from build123d import *

# Parameters (mm, degrees)
SKETCH_1_R      = 56
SKETCH_1_R_2    = 2.6
SKETCH_1_R_3    = 17.5
SKETCH_1_R_4    = 1.5
EXTRUDE_1_DEPTH = 4
FILLET_1_R      = 3
EXTRUDE_START   = -4
SKETCH_2_R      = 17.5
SKETCH_2_R_2    = 7.5
EXTRUDE_2_DEPTH = 4


with BuildPart() as part:
    # 草图1 → 凸台-拉伸1 (new body)
    with BuildSketch(Plane(origin=(0, 0, 0), x_dir=(1, 0, 0), z_dir=(0, 1, 0))):
        with Locations(Location((0, 0, 0), (0, 0, 270))):
            Circle(SKETCH_1_R)
        with BuildLine():
            Line((-5, 47.236109069), (-5, 27.041634566))
            ThreePointArc((-5, 27.041634566), (-13.75, 23.815698604), (-20.918742494, 17.850944302))
            Line((-20.918742494, 17.850944302), (-38.40767043, 27.948181554))
            ThreePointArc((-38.40767043, 27.948181554), (-23.75, 41.13620668), (-5, 47.236109069))
        make_face(mode=Mode.SUBTRACT)
        with BuildLine():
            Line((-43.40767043, 19.287927516), (-25.918742494, 9.190690264))
            ThreePointArc((-25.918742494, 9.190690264), (-27.5, 0), (-25.918742494, -9.190690264))
            Line((-25.918742494, -9.190690264), (-43.40767043, -19.287927516))
            ThreePointArc((-43.40767043, -19.287927516), (-47.5, 0), (-43.40767043, 19.287927516))
        make_face(mode=Mode.SUBTRACT)
        with BuildLine():
            Line((-38.40767043, -27.948181554), (-20.918742494, -17.850944302))
            ThreePointArc((-20.918742494, -17.850944302), (-13.75, -23.815698604), (-5, -27.041634566))
            Line((-5, -27.041634566), (-5, -47.236109069))
            ThreePointArc((-5, -47.236109069), (-23.75, -41.13620668), (-38.40767043, -27.948181554))
        make_face(mode=Mode.SUBTRACT)
        with BuildLine():
            Line((5, -47.236109069), (5, -27.041634566))
            ThreePointArc((5, -27.041634566), (13.75, -23.815698604), (20.918742494, -17.850944302))
            Line((20.918742494, -17.850944302), (38.40767043, -27.948181554))
            ThreePointArc((38.40767043, -27.948181554), (23.75, -41.13620668), (5, -47.236109069))
        make_face(mode=Mode.SUBTRACT)
        with BuildLine():
            Line((43.40767043, -19.287927516), (25.918742494, -9.190690264))
            ThreePointArc((25.918742494, -9.190690264), (27.5, 0), (25.918742494, 9.190690264))
            Line((25.918742494, 9.190690264), (43.40767043, 19.287927516))
            ThreePointArc((43.40767043, 19.287927516), (47.5, 0), (43.40767043, -19.287927516))
        make_face(mode=Mode.SUBTRACT)
        with BuildLine():
            Line((38.40767043, 27.948181554), (20.918742494, 17.850944302))
            ThreePointArc((20.918742494, 17.850944302), (13.75, 23.815698604), (5, 27.041634566))
            Line((5, 27.041634566), (5, 47.236109069))
            ThreePointArc((5, 47.236109069), (23.75, 41.13620668), (38.40767043, 27.948181554))
        make_face(mode=Mode.SUBTRACT)
        with Locations(Location((0, 22.55, 0), (0, 0, 270))):
            Circle(SKETCH_1_R_2, mode=Mode.SUBTRACT)
        with Locations(Location((-19.528872855, -11.275, 0), (0, 0, 270))):
            Circle(SKETCH_1_R_2, mode=Mode.SUBTRACT)
        with Locations(Location((0, -22.55, 0), (0, 0, 270))):
            Circle(SKETCH_1_R_2, mode=Mode.SUBTRACT)
        with Locations(Location((19.528872855, -11.275, 0), (0, 0, 270))):
            Circle(SKETCH_1_R_2, mode=Mode.SUBTRACT)
        with Locations(Location((-19.528872855, 11.275, 0), (0, 0, 270))):
            Circle(SKETCH_1_R_2, mode=Mode.SUBTRACT)
        with Locations(Location((0, 0, 0), (0, 0, 270))):
            Circle(SKETCH_1_R_3, mode=Mode.SUBTRACT)
        with Locations(Location((19.528872855, 11.275, 0), (0, 0, 270))):
            Circle(SKETCH_1_R_2, mode=Mode.SUBTRACT)
        with Locations(Location((-32.421469697, -40.655237088, 0), (0, 0, 270))):
            Circle(SKETCH_1_R_4, mode=Mode.SUBTRACT)
        with Locations(Location((-40.655237088, -32.421469697, 0), (0, 0, 270))):
            Circle(SKETCH_1_R_4, mode=Mode.SUBTRACT)
        with Locations(Location((-22.561954434, -46.850381131, 0), (0, 0, 270))):
            Circle(SKETCH_1_R_4, mode=Mode.SUBTRACT)
        with Locations(Location((-11.571088566, -50.696251433, 0), (0, 0, 270))):
            Circle(SKETCH_1_R_4, mode=Mode.SUBTRACT)
        with Locations(Location((-46.850381131, -22.561954434, 0), (0, 0, 270))):
            Circle(SKETCH_1_R_4, mode=Mode.SUBTRACT)
        with Locations(Location((-50.696251433, -11.571088566, 0), (0, 0, 270))):
            Circle(SKETCH_1_R_4, mode=Mode.SUBTRACT)
        with Locations(Location((-52, 0, 0), (0, 0, 270))):
            Circle(SKETCH_1_R_4, mode=Mode.SUBTRACT)
        with Locations(Location((0, -52, 0), (0, 0, 270))):
            Circle(SKETCH_1_R_4, mode=Mode.SUBTRACT)
        with Locations(Location((11.571088566, -50.696251433, 0), (0, 0, 270))):
            Circle(SKETCH_1_R_4, mode=Mode.SUBTRACT)
        with Locations(Location((22.561954434, -46.850381131, 0), (0, 0, 270))):
            Circle(SKETCH_1_R_4, mode=Mode.SUBTRACT)
        with Locations(Location((32.421469697, -40.655237088, 0), (0, 0, 270))):
            Circle(SKETCH_1_R_4, mode=Mode.SUBTRACT)
        with Locations(Location((40.655237088, -32.421469697, 0), (0, 0, 270))):
            Circle(SKETCH_1_R_4, mode=Mode.SUBTRACT)
        with Locations(Location((46.850381131, -22.561954434, 0), (0, 0, 270))):
            Circle(SKETCH_1_R_4, mode=Mode.SUBTRACT)
        with Locations(Location((50.696251433, -11.571088566, 0), (0, 0, 270))):
            Circle(SKETCH_1_R_4, mode=Mode.SUBTRACT)
        with Locations(Location((-50.696251433, 11.571088566, 0), (0, 0, 270))):
            Circle(SKETCH_1_R_4, mode=Mode.SUBTRACT)
        with Locations(Location((-46.850381131, 22.561954434, 0), (0, 0, 270))):
            Circle(SKETCH_1_R_4, mode=Mode.SUBTRACT)
        with Locations(Location((-40.655237088, 32.421469697, 0), (0, 0, 270))):
            Circle(SKETCH_1_R_4, mode=Mode.SUBTRACT)
        with Locations(Location((-32.421469697, 40.655237088, 0), (0, 0, 270))):
            Circle(SKETCH_1_R_4, mode=Mode.SUBTRACT)
        with Locations(Location((-22.561954434, 46.850381131, 0), (0, 0, 270))):
            Circle(SKETCH_1_R_4, mode=Mode.SUBTRACT)
        with Locations(Location((-11.571088566, 50.696251433, 0), (0, 0, 270))):
            Circle(SKETCH_1_R_4, mode=Mode.SUBTRACT)
        with Locations(Location((40.655237088, 32.421469697, 0), (0, 0, 270))):
            Circle(SKETCH_1_R_4, mode=Mode.SUBTRACT)
        with Locations(Location((22.561954434, 46.850381131, 0), (0, 0, 270))):
            Circle(SKETCH_1_R_4, mode=Mode.SUBTRACT)
        with Locations(Location((11.571088566, 50.696251433, 0), (0, 0, 270))):
            Circle(SKETCH_1_R_4, mode=Mode.SUBTRACT)
        with Locations(Location((0, 52, 0), (0, 0, 270))):
            Circle(SKETCH_1_R_4, mode=Mode.SUBTRACT)
        with Locations(Location((46.850381131, 22.561954434, 0), (0, 0, 270))):
            Circle(SKETCH_1_R_4, mode=Mode.SUBTRACT)
        with Locations(Location((32.421469697, 40.655237088, 0), (0, 0, 270))):
            Circle(SKETCH_1_R_4, mode=Mode.SUBTRACT)
        with Locations(Location((52, 0, 0), (0, 0, 270))):
            Circle(SKETCH_1_R_4, mode=Mode.SUBTRACT)
        with Locations(Location((50.696251433, 11.571088566, 0), (0, 0, 270))):
            Circle(SKETCH_1_R_4, mode=Mode.SUBTRACT)
    extrude(amount=EXTRUDE_1_DEPTH)

    # 圆角1
    fillet_1_edges = [part.edges().sort_by_distance(p)[0] for p in [
        (5, 2, 27.041634566),
        (5, 2, 47.236109069),
        (38.40767043, 2, 27.948181554),
        (20.918742494, 2, 17.850944302),
        (43.40767043, 2, -19.287927516),
        (25.918742494, 2, -9.190690264),
        (25.918742494, 2, 9.190690264),
        (43.40767043, 2, 19.287927516),
        (5, 2, -47.236109069),
        (5, 2, -27.041634566),
        (20.918742494, 2, -17.850944302),
        (38.40767043, 2, -27.948181554),
        (-38.40767043, 2, -27.948181554),
        (-20.918742494, 2, -17.850944302),
        (-5, 2, -27.041634566),
        (-5, 2, -47.236109069),
        (-43.40767043, 2, 19.287927516),
        (-25.918742494, 2, 9.190690264),
        (-25.918742494, 2, -9.190690264),
        (-43.40767043, 2, -19.287927516),
        (-5, 2, 47.236109069),
        (-5, 2, 27.041634566),
        (-20.918742494, 2, 17.850944302),
        (-38.40767043, 2, 27.948181554),
    ]]
    fillet(fillet_1_edges, radius=FILLET_1_R)

    # 草图2 → 凸台-拉伸2 (add)
    with BuildSketch(Plane(origin=(0, 4, 0), x_dir=(1, 0, 0), z_dir=(0, 1, 0)).offset(EXTRUDE_START)):
        Circle(SKETCH_2_R)
        with Locations(Location((0, 0, 0), (0, 0, 270))):
            Circle(SKETCH_2_R_2, mode=Mode.SUBTRACT)
    extrude(amount=EXTRUDE_2_DEPTH)


solid = part.part
Design review of the part built by this model. Coordinates are the model's own, in mm. Give positions to 0.01 mm unless a question says otherwise; leave off trailing zeros. Loops run counter-clockwise (first coordinate to the right, second up) from the corner with the lowest first, then second, coordinate; pieces in that order, holes last. Notation, with made-up numbers: (-0.5, 2.5) -> (47.5, 2.5) arc R15 ccw to (47.5, 30.5) -> close; hole circle Ø5 at (76, 33.25). An arc over 180 degrees is marked (long way). One line per question, with ' | ' between items. Start each with the question number.
(1) Insertion check: P1, Ø1.5, axis at y = 2, z = 3, coming from the +X side; P2, Ø1.2, axis at y = 2, z = 40, coming from the +X side (3 decimals); P3, Ø2, axis at x = -42, y = 0.5, coming from the +Z side. Each pin has a flat end and moves straight along its axis. Give the tip position at first contact, or say it passes through.
(2) For line 1 (Z direction, x = -35, y = 1.2); line 2 (Z direction, x = -2, y = 2.5); line 3 (X direction, y = 1.35, z = -5.5), list the stretches that pass through material, from the lowest coordinate up.
(3) We need section A-A (z = 0). State the section outline as (x, y) points.
(4) We need section C-C (z = -37). State the section outline as (x, y) points, and give its area (3 significant figures).
(5) We need section D-D (y = 0.6). State how many separate pieces and enclosed holes the cut face has, and give its area (3 significant figures).
(6) We need section B-B (x = 0). State the section outline as (y, z) points, and give its area (3 significant figures).
The answers:
1) P1: stops at x = 55.95 | P2: stops at x = 39.795 | P3: stops at z = 38.14
2) line 1: z = -43.71 to -32.11, -25.98 to -14.43, 14.43 to 25.98, 32.11 to 43.71 | line 2: z = -55.96 to -24.21, -20.89 to -7.23, 7.23 to 20.89, 24.21 to 55.96 | line 3: x = -55.73 to -47.18, -26.94 to -5.1, 5.1 to 26.94, 47.18 to 55.73
3) outline: (-56, 0) -> (-53.5, 0) -> (-53.5, 4) -> (-56, 4) -> close; (-50.5, 0) -> (-47.5, 0) -> (-47.5, 4) -> (-50.5, 4) -> close; (-27.5, 0) -> (-7.5, 0) -> (-7.5, 4) -> (-27.5, 4) -> close; (7.5, 0) -> (27.5, 0) -> (27.5, 4) -> (7.5, 4) -> close; (47.5, 0) -> (50.5, 0) -> (50.5, 4) -> (47.5, 4) -> close; (53.5, 0) -> (56, 0) -> (56, 4) -> (53.5, 4) -> close
4) outline: (-42.04, 0) -> (-29.79, 0) -> (-29.79, 4) -> (-42.04, 4) -> close; (-5, 0) -> (5, 0) -> (5, 4) -> (-5, 4) -> close; (29.79, 0) -> (42.04, 0) -> (42.04, 4) -> (29.79, 4) -> close | area: 138 mm^2
5) separate pieces: 1 | enclosed holes: 41 | area: 5,890 mm^2
6) outline: (0, -56) -> (4, -56) -> (4, -53.5) -> (0, -53.5) -> close; (0, -50.5) -> (4, -50.5) -> (4, -25.15) -> (0, -25.15) -> close; (0, -19.95) -> (4, -19.95) -> (4, -7.5) -> (0, -7.5) -> close; (0, 7.5) -> (4, 7.5) -> (4, 19.95) -> (0, 19.95) -> close; (0, 25.15) -> (4, 25.15) -> (4, 50.5) -> (0, 50.5) -> close; (0, 53.5) -> (4, 53.5) -> (4, 56) -> (0, 56) -> close | area: 322 mm^2
